Input: part model. Units: mm. Frame: model coordinates. A direction names the side the tool comes from. Round coordinates to 2 decimals unless told otherwise and drop trailing zeros. Order: outer loops, then holes, each group sorted by start corner. A loop starts at its lowest first (then second) coordinate and runs counter-clockwise, first axis right, second up. Notation, with made-up numbers: (35, -5.75) -> (44, -5.75) arc R27 cw to (44, 10.25) -> close; hole circle Ø9 at (9, -29). An arc over 180 degrees is marked (long way). Use a Markdown table: item, result.
Autodesk Inventor part; units mm, degrees
ref_plane "YZ Plane" through (0, 0, 0) normal (1, 0, 0) x (0, 1, 0)
ref_plane "XZ Plane" through (0, 0, 0) normal (0, 1, 0) x (-1, 0, 0)
ref_plane "XY Plane" through (0, 0, 0) normal (0, 0, 1) x (1, 0, 0)
sketch "Sketch1" plane through (0, 0, 0) normal (0, 0, 1) x (1, 0, 0)
  circle A0 centre (-39.5, 39.5) radius 1.5875
  circle A1 centre (39.5, 39.5) radius 1.5875
  circle A2 centre (39.5, -39.5) radius 1.5875
  circle A3 centre (-39.5, -39.5) radius 1.5875
  line L0 (0, 0) -> (0, 46)
  line L1 (0, 0) -> (49.2895, 0)
  line L2 (-4.4901, 16.5099) -> (-33.9803, 46)
  line L3 (4.4901, 16.5099) -> (33.9803, 46)
  line L4 (-33.9803, -46) -> (-4.4901, -16.5099)
  line L5 (4.4901, -16.5099) -> (33.9803, -46)
  line L6 (-47.625, 46) -> (-33.9803, 46)
  line L7 (33.9803, 46) -> (47.625, 46)
  line L8 (47.625, -46) -> (33.9803, -46)
  line L9 (-33.9803, -46) -> (-47.625, -46)
  arc A4 (-4.4901, 16.5099) -> (4.4901, 16.5099) centre (0, 21) ccw
  arc A5 (4.4901, -16.5099) -> (-4.4901, -16.5099) centre (0, -21) ccw
  line L10 (-47.625, 22.9803) -> (-29.1349, 4.4901)
  line L11 (-29.1349, -4.4901) -> (-47.625, -22.9803)
  line L12 (47.625, 22.9803) -> (29.1349, 4.4901)
  line L13 (29.1349, -4.4901) -> (47.625, -22.9803)
  arc A6 (-29.1349, -4.4901) -> (-29.1349, 4.4901) centre (-33.625, 0) ccw
  arc A7 (29.1349, 4.4901) -> (29.1349, -4.4901) centre (33.625, 0) ccw
  line L14 (47.625, 46) -> (47.625, 22.9803)
  line L15 (47.625, -22.9803) -> (47.625, -46)
  line L16 (-47.625, -46) -> (-47.625, -22.9803)
  line L17 (-47.625, 22.9803) -> (-47.625, 46)
  point P0 (0, 12.0197)
  point P1 (0, -12.0197)
  point P2 (-24.6447, 0)
  point P3 (24.6447, 0)
  dimension "d0" = 79
  dimension "d1" = 79
  dimension "d2" = 3.175
  dimension "d5" = 6.35
  dimension "d6" = 25
  dimension "d7" = 25
  dimension "d8" = 92
  dimension "d9" = 6.35
  dimension "d10" = 95.25
  dimension "d11" = 14
extrude "Extrusion1" add sketch "Sketch1" along normal mid plane 8.15
sketch "Sketch2" plane through (0, 0, 4.075) normal (0, 0, 1) x (1, 0, 0)
  circle A0 centre (-39.5, -39.5) radius 1.5875
  circle A1 centre (39.5, 39.5) radius 1.5875
  circle A2 centre (-39.5, 39.5) radius 1.5875
  line L0 (-33.9803, 46) -> (-47.625, 46)
  line L1 (-47.625, 46) -> (-47.625, 22.9803)
  line L2 (-47.625, -46) -> (-33.9803, -46)
  line L3 (47.625, 46) -> (33.9803, 46)
  line L4 (-33, 46) -> (-33, 33)
  line L5 (-33, 33) -> (-47.625, 33)
  line L6 (-47.625, 33) -> (-47.625, -33)
  line L7 (-47.625, -33) -> (-33, -33)
  line L8 (-33, -33) -> (-33, -46)
  line L9 (-33, -46) -> (33, -46)
  line L10 (33, -46) -> (33, -33)
  line L11 (33, -33) -> (47.625, -33)
  line L12 (47.625, -33) -> (47.625, 33)
  line L13 (47.625, 33) -> (33, 33)
  line L14 (33, 33) -> (33, 46)
  line L15 (33, 46) -> (-33, 46)
  point P0 (0, 0)
  dimension "d14" = 6.5
  dimension "d15" = 6.5
  dimension "d16" = 6.5
  dimension "d17" = 6.5
extrude "Extrusion2" cut sketch "Sketch2" against normal blind 2.45 contours L5 L4 L15 L14 L13 L12 L11 L10 L9 L8 L7 L6 L1
mirror "Mirror1" about plane through (0, 0, 0) normal (0, 0, 1) of "Extrusion2"
hole "Hole1" at (47.625, 39.5, 0) direction (-1, 0, 0) diameter 3.048 depth 5.3848 tip angle 118 countersink diameter 3.937 countersink angle 120
mirror "Mirror2" about plane through (0, 0, 0) normal (0, 1, 0) of "Hole1"
mirror "Mirror3" about plane through (0, 0, 0) normal (1, 0, 0) of "Hole1", "Mirror2"
ref_plane "Work Plane3" through (-27.275, 0, 1.625) normal (0, -1, 0) x (1, 0, 0)
ref_plane "Work Plane4" through (0, -14.65, 1.625) normal (1, 0, 0) x (0, 0, -1)
properties part number "RT-IHU_heatsink"
1) Cut plane A-A on x = -39.5. Return loops of the section in (y, z) (1 decimal).
Answer key:
| item | result |
|---|---|
| outline | (-46, -4.1) -> (-41.1, -4.1) -> (-41.1, 4.1) -> (-46, 4.1) -> close; (-37.9, -4.1) -> (-33, -4.1) -> (-33, -1.6) -> (-14.9, -1.6) -> (-14.9, 1.6) -> (-33, 1.6) -> (-33, 4.1) -> (-37.9, 4.1) -> close; (14.9, -1.6) -> (33, -1.6) -> (33, -4.1) -> (37.9, -4.1) -> (37.9, 4.1) -> (33, 4.1) -> (33, 1.6) -> (14.9, 1.6) -> close; (41.1, -4.1) -> (46, -4.1) -> (46, 4.1) -> (41.1, 4.1) -> close |
2) Contact query for flat-ended pins moving along their axis: P1, Ø10, axis at x = 18, y = 3.5, coming from the +Z side (3 decimals); P2, Ø4, axis at x = -39.5, y = -39.5, coming from the -Z side (3 decimals); P3, Ø4, axis at y = 4, z = 1.5, coming from the -X side; P4, Ø2, axis at x = 3.5, z = -1.5, coming from the -Y side. Output: stop coordinate, or through.
Answer key:
| item | result |
|---|---|
| P1 | stops at z = 1.625 |
| P2 | stops at z = -4.075 |
| P3 | stops at x = -30.64 |
| P4 | stops at y = -16.52 |
3) Cut plane D-D on x = 11. Return loops of the section in (y, z) (3 decimals), and give its area (3 significant figures).
Answer key:
| item | result |
|---|---|
| outline | (-23.02, -1.625) -> (23.02, -1.625) -> (23.02, 1.625) -> (-23.02, 1.625) -> close |
| area | 150 mm^2 |
4) Cut plane C-C on y = -28. Return loops of the section in (x, z) (3 decimals), and give its area (3 significant figures).
Answer key:
| item | result |
|---|---|
| outline | (-47.625, -1.625) -> (-15.98, -1.625) -> (-15.98, 1.625) -> (-47.625, 1.625) -> close; (15.98, -1.625) -> (47.625, -1.625) -> (47.625, 1.625) -> (15.98, 1.625) -> close |
| area | 206 mm^2 |
5) Ray query, probe 1 along X at (y, z) = (-39, 3.75) (3 decimals); probe 2 along Y at (x, z) = (-39.5, 1.5); probe 3 along Y at (x, z) = (34, 3). Return the intervals inside material, ascending.
Answer key:
| item | result |
|---|---|
| probe 1 | x = -47.625 to -41.007, -37.993 to -33, 33 to 37.993, 41.007 to 47.625 |
| probe 2 | y = -46 to -41.09, -37.91 to -14.86, 14.86 to 37.91, 41.09 to 46 |
| probe 3 | y = -46 to -33, 33 to 46 |
6) Cut plane B-B on y = 31. Return loops of the section in (x, z) (3 decimals), and give its area (3 significant figures).
Answer key:
| item | result |
|---|---|
| outline | (-47.625, -1.625) -> (-18.98, -1.625) -> (-18.98, 1.625) -> (-47.625, 1.625) -> close; (18.98, -1.625) -> (47.625, -1.625) -> (47.625, 1.625) -> (18.98, 1.625) -> close |
| area | 186 mm^2 |
7) Set-up query: faces 4 (the face through (-40, -33, -3)), 5 (the face through (-33, -39, 3)), 6 (the face through (-38.509, 13.865, -0.023)), 7 (the face through (-33, -39, -3)), 8 (the face through (44.768, 38.215, -0.819)). Return all of +Z, -Z, +X, -X, +Y, -Y with unobstructed straight access to the full face (end or side cutting, diameter ignored); none if empty.
Answer key:
| item | result |
|---|---|
| face 4 | -Z, +X, -X |
| face 5 | +Z, +Y, -Y |
| face 6 | +Z, -Z, -X |
| face 7 | -Z, +Y, -Y |
| face 8 | +X |
8) Draft query along Z for faces 1 (the face through (-20.26, 32.28, -0.62)), 2 (the face through (41.484, -39.758, 0.057)), 3 (the face through (-40.4, -38, 4.075)). Return one class per face: released by +Z, released by -Z, zero draft, split by the parting line, or undercut.
Answer key:
| item | result |
|---|---|
| face 1 | zero draft |
| face 2 | undercut |
| face 3 | released by +Z |
